CAD build for the part. Positions are in the model's coordinates, mm. A direction names the side the tool comes from. Round coordinates to 2 decimals unless told otherwise and drop trailing zeros. Loops run counter-clockwise (first coordinate to the right, second up) from the corner with the lowest first, then second, coordinate; pieces in that order, holes last.
```python
from build123d import *

# Parameters (mm, degrees)
SKETCH_1_W      = 12
SKETCH_1_H      = 12
SKETCH_1_R      = 1
SKETCH_1_W_2    = 5
EXTRUDE_1_DEPTH = 2
SKETCH_2_W      = 17
SKETCH_2_H      = 2.2
EXTRUDE_2_DEPTH = 2.5
EXTRUDE_3_DEPTH = 17
CHAMFER_1_SIZE  = 1
FILLET_4_R      = 2


with BuildPart() as part:
    # 草图1 → 凸台-拉伸1 (new body)
    # profile 1 of 2: a face of its own
    with BuildSketch(Plane(origin=(0, 0, 0), x_dir=(1, 0, 0), z_dir=(0, 1, 0))):
        Rectangle(SKETCH_1_W, SKETCH_1_H)
        with Locations(Location((2.5, 0, 0), (0, 0, 270))):
            Circle(SKETCH_1_R, mode=Mode.SUBTRACT)
        with Locations(Location((-2.5, 0, 0), (0, 0, 270))):
            Circle(SKETCH_1_R, mode=Mode.SUBTRACT)
    # profile 2 of 2: a face of its own
    with BuildSketch(Plane(origin=(0, 0, 0), x_dir=(1, 0, 0), z_dir=(0, 1, 0))):
        with Locations((-8.5, 0)):
            Rectangle(SKETCH_1_W_2, SKETCH_1_H)
    extrude(amount=EXTRUDE_1_DEPTH)

    # 草图2 → 凸台-拉伸2 (add)
    with BuildSketch(Plane(origin=(0, 2, 0), x_dir=(1, 0, 0), z_dir=(0, 1, 0))):
        with Locations((-2.5, 4.9)):
            Rectangle(SKETCH_2_W, SKETCH_2_H)
        with Locations((-2.5, -4.9)):
            Rectangle(SKETCH_2_W, SKETCH_2_H)
    extrude(amount=EXTRUDE_2_DEPTH)

    # 草图4 → 凸台-拉伸3 (add)
    with BuildSketch(Plane(origin=(6, 0, 0), x_dir=(0, 0, -1), z_dir=(1, 0, 0))):
        with BuildLine():
            Line((-6, 5.5), (-6, 4.5))
            Line((-6, 4.5), (6, 4.5))
            Line((6, 4.5), (6, 5.5))
            Line((6, 5.5), (4.227921486, 8.030790397))
            ThreePointArc((4.227921486, 8.030790397), (0, 15.7), (-4.227921486, 8.030790397))
            Line((-4.227921486, 8.030790397), (-6, 5.5))
        make_face()
        with BuildLine():
            ThreePointArc((0, 7.85), (-2.85, 10.7), (0, 13.55))
            ThreePointArc((0, 13.55), (2.85, 10.7), (0, 7.85))
        make_face(mode=Mode.SUBTRACT)
    extrude(amount=-EXTRUDE_3_DEPTH)

    # 圆角1: read off the stored shape, not the designer's step
    # 圆角1 outline → 圆角1 (revolve, cut)
    with BuildSketch(Plane(origin=(0, 10.7, 0), x_dir=(0, 1, 0), z_dir=(0, 0, -1))):
        with BuildLine():
            Line((2.85, 6), (2.85, 5.5))
            ThreePointArc((2.85, 5.5), (2.996446609, 5.853553391), (3.35, 6))
            Line((3.35, 6), (2.85, 6))
        make_face()
        with BuildLine():
            ThreePointArc((3.35, -11), (2.996446609, -10.853553391), (2.85, -10.5))
            Line((2.85, -10.5), (2.85, -11))
            Line((2.85, -11), (3.35, -11))
        make_face()
    revolve(axis=Axis((0, 10.7, 0), (1, 0, 0)), mode=Mode.SUBTRACT)

    # 倒角1
    chamfer_1_edges = [part.edges().sort_by_distance(p)[0] for p in [
        (6, 0, 0),
    ]]
    chamfer(chamfer_1_edges, length=CHAMFER_1_SIZE)

    # 圆角4
    fillet_4_edges = [part.edges().sort_by_distance(p)[0] for p in [
        (-3, 0, -6),
        (-3, 0, 6),
    ]]
    fillet(fillet_4_edges, radius=FILLET_4_R)


solid = part.part
```
Item 1: Cut at D-D, the plane x = 1. Give the cut face in (y, z).
Answers follow:
outline: (0, -4) arc R2 ccw to (2, -6) - (5.5, -6) - (8.03, -4.23) arc R5 ccw (long way) to (8.03, 4.23) - (5.5, 6) - (2, 6) arc R2 ccw to (0, 4) - close; hole (2, -3.8) - (4.5, -3.8) - (4.5, 3.8) - (2, 3.8) - close; hole circle Ø5.7 at (10.7, 0)
Item 2: Cut at C-C, the plane z = 0. Give the cut face in (x, y).
Answers follow:
outline: (-11, 0) - (-3.5, 0) - (-3.5, 2) - (-11, 2) - close; (-11, 4.5) - (6, 4.5) - (6, 7.35) arc R0.5 ccw to (5.5, 7.85) - (-10.5, 7.85) arc R0.5 ccw to (-11, 7.35) - close; (-11, 14.05) arc R0.5 ccw to (-10.5, 13.55) - (5.5, 13.55) arc R0.5 ccw to (6, 14.05) - (6, 15.7) - (-11, 15.7) - close; (-1.5, 0) - (1.5, 0) - (1.5, 2) - (-1.5, 2) - close; (3.5, 0) - (5, 0) - (6, 1) - (6, 2) - (3.5, 2) - close
Item 3: Flat gauge pins, fed straight in: P1, Ø8, axis at x = 0, y = 11, coming from the +Z side; P2, Ø3, axis at x = -3.5, y = 13.5, coming from the -Z side. Where does each tip first touch, or does it go through?
Answers follow:
P1: stops at z = 5
P2: stops at z = -4.83
Item 4: 3-axis set-ups, long thin cutter, end or side, ignore diameter. For faces 1 (the flat face through (-2.381, 6.783, 5.102)), 2 (the flat face through (-11, 6, 0)), 3 (the cylindrical face through (3.49, 0.99, -0.13)), 4 (the flat face through (-2.381, 6.748, -5.126)), 5 (the flat face through (-2, 4.5, 0)): which of +Z, -Z, +X, -X, +Y, -Y reach the whole face in a straight line?
Answers follow:
face 1: +Z, +X, -X
face 2: +Z, -Z, -X, +Y, -Y
face 3: -Y
face 4: -Z, +X, -X
face 5: +X, -X
Item 5: Probe line 1 (X direction, y = 1.2, z = 0); line 2 (Y direction, x = -1.5, z = -2); line 3 (Y direction, x = -9, z = 2.5). List the from-to ranges inside material, lowest first.
Answers follow:
line 1: x = -11 to -3.5, -1.5 to 1.5, 3.5 to 6
line 2: y = 0 to 2, 4.5 to 8.67, 12.73 to 15.28
line 3: y = 0 to 2, 4.5 to 9.33, 12.07 to 15.03
Item 6: Two-plate mould, pull along Z, no slides. Class faces 6 (the flat face through (-5, 0, 0)), 7 (the cylindrical face through (-2.62, 0.57, -5.4)), 8 (the flat face through (-3, 2, -2)): released by +Z, released by -Z, zero draft, split by the parting line, or undercut.
Answers follow:
face 6: zero draft
face 7: released by -Z
face 8: undercut
Item 7: Cut at B-B, the plane x = -2.5. Give the cut face in (y, z), plus the area to 3 significant figures.
Answers follow:
outline: (0, -4) arc R2 ccw to (2, -6) - (5.5, -6) - (8.03, -4.23) arc R5 ccw (long way) to (8.03, 4.23) - (5.5, 6) - (2, 6) arc R2 ccw to (0, 4) - (0, 1) - (2, 1) - (2, 3.8) - (4.5, 3.8) - (4.5, -3.8) - (2, -3.8) - (2, -1) - (0, -1) - close; hole circle Ø5.7 at (10.7, 0)
area: 106 mm2
Item 8: Cut at A-A, the plane y = 10.7. Give the cut face in (x, z), plus the area to 3 significant figures.
Answers follow:
outline: (-11, -5) - (6, -5) - (6, -3.35) arc R0.5 ccw to (5.5, -2.85) - (-10.5, -2.85) arc R0.5 ccw to (-11, -3.35) - close; (-11, 3.35) arc R0.5 ccw to (-10.5, 2.85) - (5.5, 2.85) arc R0.5 ccw to (6, 3.35) - (6, 5) - (-11, 5) - close
area: 72.9 mm2
